Work out the finished part from the listing and answer in its coordinate system (mm). Face numbers are marked on the shaded views. A direction names the side the tool comes from. Give positions to 0.01 mm unless a question says otherwise; leave off trailing zeros. Write each loop counter-clockwise with the first axis right and the second up, starting at its lowest first coordinate (ties: lowest second). Pieces come first, ordered by that corner, then holes.
1) A tool of negligible diameter and unlimited length cuts with its end or side. For the marked faces 1, 2 and 3, from which of +Z, -Z, +X, -X, +Y, -Y can it reach the whole face along a straight path? Write none if from no direction.
2) Find section B-B (x = 2.5). Determine the outline of the cut face in (y, z), plus the area to 3 significant figures.
3) Find section A-A (z = 9). Determine the outline of the cut face in (x, y) (3 decimals).
4) Straight lines are drawn through the part: probe 1 along X at (y, z) = (5, 57.5); probe 2 along Z at (x, y) = (12.75, 7); probe 3 along Y at (x, z) = (14.75, -8). For each, find the intervals that lie inside material, in ascending order.
5) Given pin 1 Ø3 at (x, z) = (8, 24.5) entering from +Y; pin 2 Ø7.5 at (x, z) = (3.5, 88) entering from -Y; pin 3 Ø2 at (y, z) = (11, -11) entering from +X, each flat-ended and moving along its own axis, determine where each tip first touches the part or whether it passes through.
6) Find section D-D (z = 83.5). Determine the outline of the cut face in (x, y), plus the area to 3 significant figures.
7) Find section C-C (y = -2). Determine the outline of the cut face in (x, z) (3 decimals).
```python
from build123d import *

# Parameters (mm, degrees)
BOSS_EXTRUDE1_DEPTH = 12.7
BOSS_EXTRUDE2_DEPTH = 3.175


with BuildPart() as part:
    # Sketch1 → Boss-Extrude1 (new, symmetric)
    with BuildSketch(Plane(origin=(0, 0, 0), x_dir=(0, 0, -1), z_dir=(1, 0, 0))):
        Polygon((-68.297268412, 0), (-41.236086589, 18.224877555), (32.952051336, 18.224877555), (47.679225118, 1.472717378), (32.952051336, -17.488518866), (-33.136141009, -17.488518866), (-68.297268412, -4.234062462), (-117.449210909, -4.234062462), (-117.449210909, 1.472717378), align=None)
    extrude(amount=BOSS_EXTRUDE1_DEPTH, both=True)

    # Sketch2 → Boss-Extrude2 (add)
    with BuildSketch(Plane(origin=(12.7, 0, 0), x_dir=(0, 0, -1), z_dir=(1, 0, 0))):
        Polygon((-29.747162431, -17.985294415), (24.617608562, -13.228993258), (21.600184439, 21.260322286), (-32.764586554, 16.504021128), align=None)
        Polygon((-24.177392815, 5.781642489), (-17.851556482, 6.335081455), (-18.404995449, 12.660917788), (-24.730831781, 12.107478822), align=None, mode=Mode.SUBTRACT)
        Polygon((7.451788849, 8.548837321), (13.777625182, 9.102276288), (13.224186216, 15.428112621), (6.898349883, 14.874673654), align=None, mode=Mode.SUBTRACT)
    extrude(amount=BOSS_EXTRUDE2_DEPTH)


solid = part.part
```
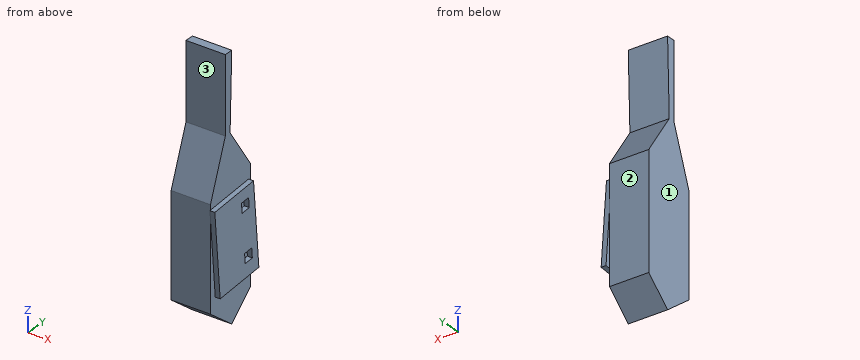
Results:
1. face 1: +Z, -Z, -X, +Y, -Y
1. face 2: +Z, -Z, -X, +Y
1. face 3: +Z, +X, -X, -Y
2. outline: (-17.49, -32.95) - (1.47, -47.68) - (18.22, -32.95) - (18.22, 41.24) - (0, 68.3) - (1.47, 117.45) - (-4.23, 117.45) - (-4.23, 68.3) - (-17.49, 33.14) - close
2. area: 3,640 mm2
3. outline: (-12.7, -17.489) - (12.7, -17.489) - (12.7, -16.17) - (15.875, -16.17) - (15.875, 18.583) - (12.7, 18.583) - (12.7, 18.225) - (-12.7, 18.225) - close
4. probe 1: x = -12.7 to 12.7
4. probe 2: z = -22.85 to 17.91, 24.28 to 31.93
4. probe 3: y = -14.68 to 8.6, 14.97 to 20.07
5. pin 1: stops at y = 18.22
5. pin 2: stops at y = -4.23
5. pin 3: stops at x = 12.7
6. outline: (-12.7, -4.23) - (12.7, -4.23) - (12.7, 0.46) - (-12.7, 0.46) - close
6. area: 119 mm2
7. outline: (-12.7, -44.982) - (12.7, -44.982) - (12.7, -23.635) - (15.875, -23.635) - (15.875, 31.146) - (12.7, 31.146) - (12.7, 117.449) - (-12.7, 117.449) - close
